The listing builds one solid part. Answer for the finished solid, in the listing's coordinates (mm). A direction names the side the tool comes from. Coordinates: 2 decimals unless noted, no trailing zeros. Order: outer loops, then holes, each group sorted by start corner. A loop starts at its lowest first (then second) coordinate and runs counter-clockwise, first axis right, second up. Notation, with made-up numbers: (82.5, 79) -> (119.5, 79) arc R9 cw to (119.5, 83) -> close; hole circle Ø11 at (82, 27). An arc over 180 degrees is marked (long way). Answer in a Markdown table with one row per item. Add a question column.
```python
from build123d import *

# Parameters (mm, degrees)
BOX161_W               = 0.8
BOX161_H               = 18
BOX161_DEPTH           = 0.8
BOX162_W               = 0.8
BOX162_H               = 18
BOX162_DEPTH           = 0.8
CUT084_PLACEMENT_ANGLE = 213


with BuildPart() as cubo161:
    # Box161 → Box161 (new body)
    with BuildSketch(Plane.XY):
        with Locations((0.4, 9)):
            Rectangle(BOX161_W, BOX161_H)
    extrude(amount=BOX161_DEPTH)


with BuildPart() as obj1:
    # Box162 → Box162 (new body)
    with BuildSketch(Plane(origin=(0.3, 0, 0.3), x_dir=(1, 0, 0), z_dir=(0, 0, 1))):
        with Locations((0.4, 9)):
            Rectangle(BOX162_W, BOX162_H)
    extrude(amount=BOX162_DEPTH)

    # Cut084: cut Cubo161
    add(cubo161.part, mode=Mode.SUBTRACT)


with BuildPart() as obj1_1:
    # Cut084 placement: moved
    add(obj1.part.moved(Location((-213.5, 93.2, -1.45))).rotate(Axis((-213.5, 93.2, -1.45), (0, 0, 1)), CUT084_PLACEMENT_ANGLE))


solid = obj1_1.part
```
Q1. A cutting plane is placed at A-A (x = -211.5). Determine the outline of the cut face in (y, z), then the cut area to 3 significant figures.
Q2. Straight lines are drawn through the part: line 1 (X direction, y = 81.25, z = -1.05); line 2 (X direction, y = 82.75, z = -0.85); line 3 (Y direction, x = -210.5, z = -0.9). For each, find the intervals that lie inside material, in ascending order.
Q3. A cutting plane is placed at C-C (y = 83.5). Determine the outline of the cut face in (x, z).
Q4. For faces 1 (the face through (-209, 85, -0.35)), 2 (the face through (-209, 85.2, -0.65)), determine the directions among +Z, -Z, +X, -X, +Y, -Y from which every point of the face is accessible in a straight line to the end or side of a thin tool.
Q5. Given pin 1 (1 mm diameter, centred on x = -210, y = 83.5, fed in from -Z), flat-ended and moving along its own axis, determine where the tip first touches the part or whether it passes through.
Q6. A cutting plane is placed at B-B (z = -0.5). Determine the outline of the cut face in (x, y).
Returned:
| question | item | result |
|---|---|---|
| 1 | outline | (88.1, -1.15) -> (88.65, -1.15) -> (88.65, -0.65) -> (89.57, -0.65) -> (89.57, -0.35) -> (88.1, -0.35) -> close |
| 1 | area | 0.716 mm² |
| 2 | line 1 | x = -207.05 to -206.69 |
| 2 | line 2 | x = -208.03 to -207.67 |
| 2 | line 3 | y = 86.56 to 87.11 |
| 3 | outline | (-208.51, -1.15) -> (-208.15, -1.15) -> (-208.15, -0.65) -> (-207.56, -0.65) -> (-207.56, -0.35) -> (-208.51, -0.35) -> close |
| 4 | face 1 | +Z, +X, -X, +Y, -Y |
| 4 | face 2 | -Z, +X, +Y |
| 5 | pin 1 | passes through |
| 6 | outline | (-214.42, 92.6) -> (-204.62, 77.5) -> (-203.95, 77.94) -> (-213.75, 93.04) -> close |
